Job drawing, mm, ordinate dimensions from the low corner. One solid piece. A direction names the side the tool comes from. Round coordinates to 2 decimals unless told otherwise and drop trailing zeros. Loops run counter-clockwise (first coordinate to the right, second up) from the corner with the lowest first, then second, coordinate; pieces in that order, holes last. Notation, with made-up numbers: M 74,7 L 92,7 A27 cw 92,29 Z; hole C 82.5,-27 d11. An arc over 180 degrees is marked long. One line per item, written item: value.
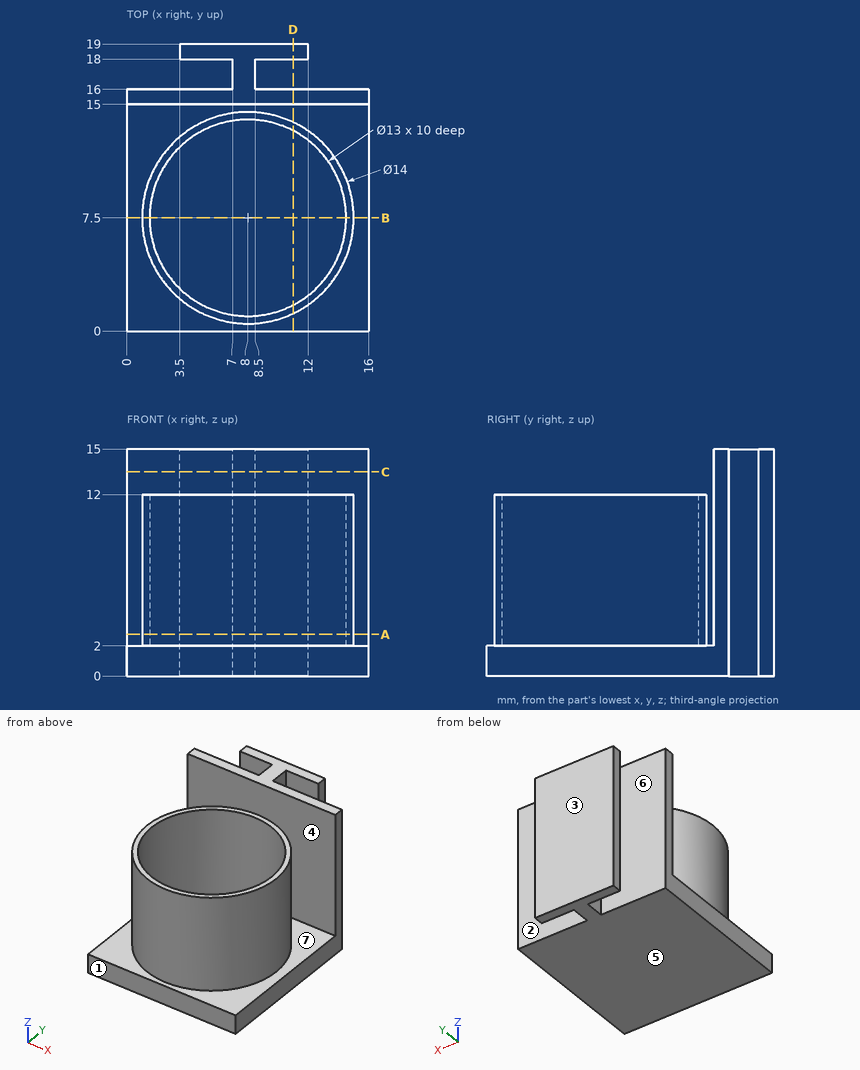
Item 1: Slice it at D-D, the plane x = 11. Give the cut face in (y, z), and give its area (3 significant figures).
Check values:
outline: M 0,0 L 16,0 L 16,15 L 15,15 L 15,2 L 13.82,2 L 13.82,12 L 13.27,12 L 13.27,2 L 1.73,2 L 1.73,12 L 1.18,12 L 1.18,2 L 0,2 Z; M 18,0 L 19,0 L 19,15 L 18,15 Z
area: 71.2 mm2
Item 2: Slice it at C-C, the plane z = 13.5. Give the cut face in (x, y), and give its area (3 significant figures).
Check values:
outline: M 0,15 L 16,15 L 16,16 L 8.5,16 L 8.5,18 L 12,18 L 12,19 L 3.5,19 L 3.5,18 L 7,18 L 7,16 L 0,16 Z
area: 27.5 mm2
Item 3: Wall check: line 1 along Y through (x, z) = (8, 8); line 2 along Y through (x, z) = (10, 1.5); line 3 along Z through (x, y) = (14.5, 1). Give the ranges that are in metal, low to high.
Check values:
line 1: y = 0.5 to 1, 14 to 14.5, 15 to 19
line 2: y = 0 to 16, 18 to 19
line 3: z = 0 to 2
Item 4: Slice it at B-B, the plane y = 7.5. Give the cut face in (x, z), and give its area (3 significant figures).
Check values:
outline: M 0,0 L 16,0 L 16,2 L 15,2 L 15,12 L 14.5,12 L 14.5,2 L 1.5,2 L 1.5,12 L 1,12 L 1,2 L 0,2 Z
area: 42.0 mm2
Item 5: Pull direction Y, two halves, no side cores. Call the marked faces 1, 2 and 3: pulls with the +Y half, pulls with the -Y half, needs draft (parallel to the pull), parting line crosses it, or undercut.
Check values:
face 1: pulls with the -Y half
face 2: undercut
face 3: pulls with the +Y half
Item 6: Which spindle directions (+Z, -Z, +X, -X, +Y, -Y) get a long thin tool onto all of the face, cutting with end or side? Do the marked faces 4, 5, 6 and 7. Say none if no direction does.
Check values:
face 4: +Z, +X, -X
face 5: -Z, +X, -X, +Y, -Y
face 6: +Z, -Z, -X
face 7: +Z
Item 7: Slice it at A-A, the plane z = 2.75. Give the cut face in (x, y), and give its area (3 significant figures).
Check values:
outline: M 0,15 L 16,15 L 16,16 L 8.5,16 L 8.5,18 L 12,18 L 12,19 L 3.5,19 L 3.5,18 L 7,18 L 7,16 L 0,16 Z; C 8,7.5 d14; hole C 8,7.5 d13
area: 48.7 mm2
Item 8: Drop flat-ended pins along their axis: P1, Ø8, axis at x = 8, y = 7.5, coming from the +Z side; P2, Ø5, axis at y = 8, z = 7, coming from the -X side; P3, Ø4, axis at x = 5, z = 8, coming from the -Y side. Give the stop position or say it passes through.
Check values:
P1: stops at z = 2
P2: stops at x = 1
P3: stops at y = 0.57
